Work out the finished part from the listing and answer in its coordinate system (mm). A direction names the side the tool comes from. Coordinates: 2 decimals unless noted, no trailing zeros. Order: outer loops, then holes, each group sorted by start corner. A loop starts at its lowest first (then second) coordinate and runs counter-clockwise, first axis right, second up.
1. A tool of negligible diameter and unlimited length cuts with its end or side. For faces 1 (the flat face through (-24, 2, -4)), 2 (the cylindrical face through (-14, 9, -8)), 3 (the flat face through (-16.5, 7, -8)), 4 (the flat face through (-11, 7, -6.5)), 5 (the flat face through (-7.5, 7, -8)), from which of +Z, -Z, +X, -X, +Y, -Y can it reach the whole face along a straight path? Write none if from no direction.
2. The part is cut by section B-B, the plane z = -4.5. Give the vertices of the cut face in (x, y).
3. Flat-ended cylindrical pins translate along their axes: pin 1 Ø3.5 at (x, z) = (-4, -4.5) entering from +Y; pin 2 Ø8 at (x, y) = (-17.5, 7.5) entering from +Z; pin 3 Ø0.8 at (y, z) = (6, -7.5) entering from -X; pin 4 Ø6.5 at (x, y) = (-12, 9) entering from +Z. Find the tip coordinate at first contact, or state that the pin passes through.
4. The part is cut by section A-A, the plane x = -12. Give the vertices of the cut face in (y, z).
5. Determine the mould class of faces 6 (the cylindrical face through (-5.01, 2.22, -5.61)), 7 (the flat face through (-12, 4.5, -4)), 8 (the cylindrical face through (-14, 9, -2)) for opening direction Y: +Y half, -Y half, draft (parallel to the pull), parting line (faces both ways), or undercut.
6. The part is cut by section C-C, the plane x = -20. Give the vertices of the cut face in (y, z), then the cut area to 3 significant figures.
7. Find the intervals of material crossed by probe 1 along X at (y, z) = (1.55, -4.5); probe 2 along X at (y, z) = (9, -7.9); probe 3 along Z at (x, y) = (-4, 1.95), in increasing order.
8. The part is cut by section D-D, the plane z = -8.25. Give the vertices of the cut face in (x, y), then the cut area to 3 significant figures.
Autodesk Inventor part; units mm, degrees
ref_plane "Plano de trabajo1" through (0, 13.5, 0) normal (0, 1, 0) x (-1, 0, 0)
ref_plane "YZ Plane" through (0, 0, 0) normal (1, 0, 0) x (0, 1, 0)
ref_plane "XY Plane" through (0, 0, 0) normal (0, 0, 1) x (1, 0, 0)
sketch "Boceto1" plane through (0, 0, 0) normal (0, 0, 1) x (1, 0, 0)
  line L0 (0, 0) -> (-24, 0)
  line L1 (-24, 0) -> (-24, 4)
  line L2 (-23.5, 4.5) -> (-0.5, 4.5)
  line L3 (0, 4) -> (0, 0)
  arc A0 (-23.5, 4.5) -> (-24, 4) centre (-23.5, 4) ccw
  arc A1 (0, 4) -> (-0.5, 4.5) centre (-0.5, 4) ccw
  line L4 (-12, 0) -> (-12, 13.5) construction
  circle A2 centre (-12, 9) radius 2
  arc A3 (-7.5, 9) -> (-16.5, 9) centre (-12, 9) ccw
  line L5 (-16.5, 9) -> (-16.5, 5)
  line L6 (-7.5, 9) -> (-7.5, 5)
  arc A4 (-17, 4.5) -> (-16.5, 5) centre (-17, 5) ccw
  arc A5 (-7.5, 5) -> (-7, 4.5) centre (-7, 5) ccw
  dimension "d0" = 24
  dimension "d2" = 1
  dimension "d3" = 1
  dimension "d4" = 4.5
  dimension "d5" = 4.5
  dimension "d6" = 4
  dimension "d7" = 9
  dimension "d8" = 1
  dimension "d9" = 1
extrude "Extrusión1" add sketch "Boceto1" against normal blind 9 contours L0 L1 A0 L2 A1 L3 | L2 A4 L5 A3 L6 A5 | A2
ref_plane "Plano de trabajo1" through (0, 13.5, 0) normal (0, 1, 0) x (-1, 0, 0)
sketch "Boceto2" plane through (0, 13.5, 0) normal (0, 1, 0) x (-1, 0, 0)
  line L0 (24, 0) -> (24, -9)
  line L1 (24, -4.5) -> (0, -4.5) construction
  line L2 (0, 0) -> (0, -9)
  line L3 (7.5, -9) -> (16.5, -9)
  line L4 (12, -9) -> (12, 0) construction
  line L5 (24, -6.5) -> (0, -6.5)
  line L6 (0, -6.5) -> (0, -2.5)
  line L7 (0, -2.5) -> (24, -2.5)
  line L8 (24, -2.5) -> (24, -6.5)
  circle A0 centre (20, -4.5) radius 1.5
  circle A1 centre (4, -4.5) radius 1.5
  point P0 (0, -4.5)
  point P1 (12, -6.5)
  point P2 (0, -6.5)
  dimension "d13" = 2
  dimension "d14" = 8
  dimension "d15" = 8
  dimension "d16" = 3
  dimension "d17" = 3
extrude "Extrusión2" cut sketch "Boceto2" against normal blind 9
hole "Agujero1" at (-20, 13.5, -4.5) at (-4, 13.5, -4.5) direction (0, -1, 0) diameter 3 end through all
hole "Agujero2" at (-12, 9, 0) direction (0, 0, -1) diameter 4 end through all countersink diameter 7 countersink angle 90
thread "Rosca1"
equation "\"d15\" = d14"
properties part number "Hudson 1-72"
Geometry says:
1. face 1: +Z, -Z, -X, +Y, -Y
1. face 2: +Z, -Z
1. face 3: +Z, -Z, -X, +Y
1. face 4: +X, -X, +Y
1. face 5: +Z, -Z, +X, +Y
2. outline: (-24, 0) - (-21.5, 0) - (-21.5, 4.5) - (-23.5, 4.5) arc R0.5 ccw to (-24, 4) - close; (-18.5, 0) - (-5.5, 0) - (-5.5, 4.5) - (-18.5, 4.5) - close; (-2.5, 0) - (0, 0) - (0, 4) arc R0.5 ccw to (-0.5, 4.5) - (-2.5, 4.5) - close
3. pin 1: stops at y = 4.5
3. pin 2: stops at z = 0
3. pin 3: stops at x = -16.5
3. pin 4: stops at z = -0.25
4. outline: (0, -9) - (7, -9) - (7, -6.5) - (4.5, -6.5) - (4.5, -2.5) - (7, -2.5) - (7, -1.5) - (5.5, 0) - (0, 0) - close; (11, -9) - (13.5, -9) - (13.5, -6.5) - (11, -6.5) - close; (11, -2.5) - (13.5, -2.5) - (13.5, 0) - (12.5, 0) - (11, -1.5) - close
5. face 6: draft
5. face 7: +Y half
5. face 8: undercut
6. outline: (0, -9) - (4.5, -9) - (4.5, -6) - (0, -6) - close; (0, -3) - (4.5, -3) - (4.5, 0) - (0, 0) - close
6. area: 27.0 mm2
7. probe 1: x = -24 to -21.5, -18.5 to -5.5, -2.5 to 0
7. probe 2: x = -16.5 to -14, -10 to -7.5
7. probe 3: z = -9 to -6, -3 to 0
8. outline: (-24, 0) - (0, 0) - (0, 4) arc R0.5 ccw to (-0.5, 4.5) - (-7, 4.5) arc R0.5 cw to (-7.5, 5) - (-7.5, 9) arc R4.5 ccw to (-16.5, 9) - (-16.5, 5) arc R0.5 cw to (-17, 4.5) - (-23.5, 4.5) arc R0.5 ccw to (-24, 4) - close; hole circle Ø4 at (-12, 9)
8. area: 168 mm2
